Here's the drawing with two shaded views (mm, measured from the low corner). I have some questions. Coordinates: 2 decimals unless noted, no trailing zeros. Write each loop counter-clockwise with the first axis right and the second up, starting at its lowest first coordinate (ties: lowest second). Pieces come first, ordered by that corner, then holes. Notation, with made-up numbers: (7.25, -27.75) - (52.25, -27.75) arc R10 ccw to (52.25, -9.75) - close; hole circle Ø10 at (19, 87.25). An arc over 180 degrees is marked (long way). Answer in a Markdown table with one row per item. Add a question column.
Item 1: Imagine slicing it at A-A (x = 12.5). Please give me the cut outline in (y, z).
Item 2: If I drill on probe 1 along X at (y, z) = (1.5, 10); probe 2 along X at (y, z) = (4, 12.5); probe 3 along X at (y, z) = (1.25, 11.75), over which ranges is the centre line in solid material (lowest first)? Write a range as from..to.
Item 3: Imagine slicing it at C-C (z = 17.5). Please give me the cut outline in (x, y).
Item 4: We'd pull the mould along Z, two halves only. Please class the marked faces 1, 2 and 3: +Z half, -Z half, draft (parallel to the pull), parting line (faces both ways), or undercut.
Item 5: Imagine slicing it at D-D (y = 6.5). Please give me the cut outline in (x, z).
Item 6: I'm going to push a flat-ended pin straight in: pin 1 (2.5 mm diameter, centred on y = 5.5, z = 9.5, fed in from -X). Where does the tip first touch, or does it pass through?
Item 7: Imagine slicing it at B-B (z = 21.75). Please give me the cut outline in (x, y), plus the area to 3 significant figures.
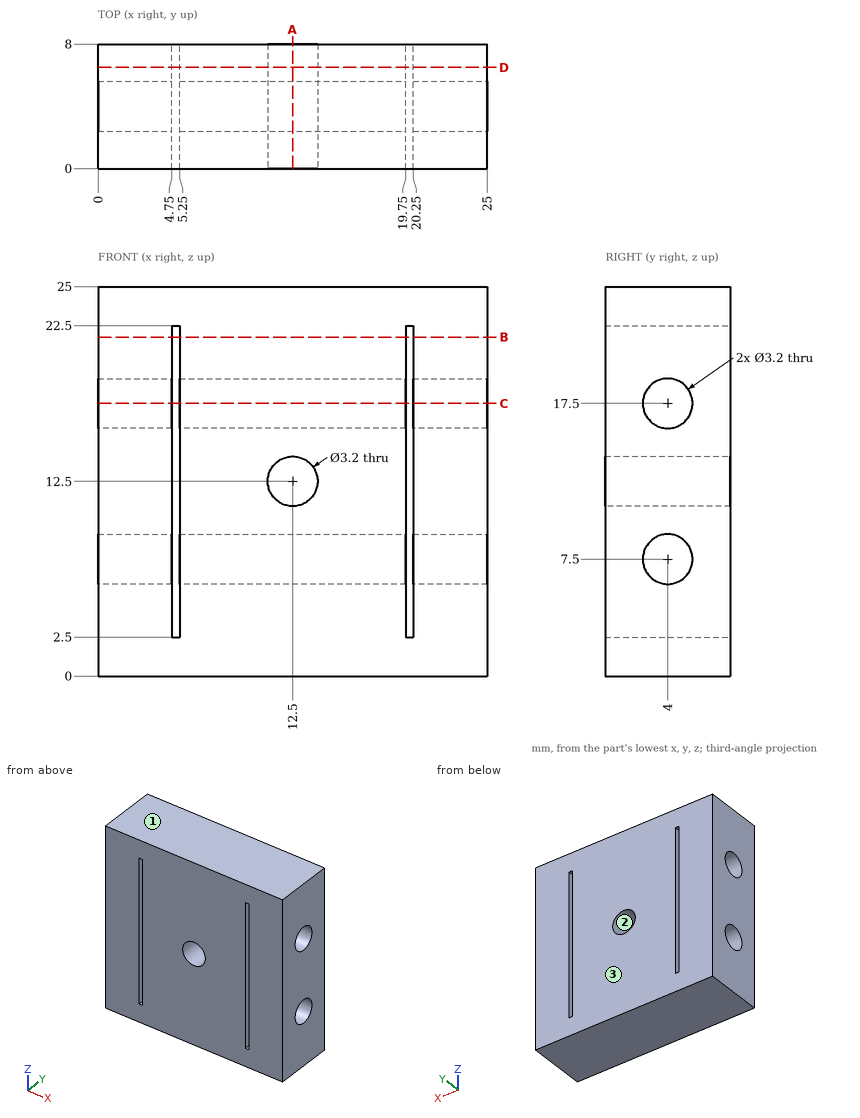
Here are the results:
| question | item | result |
|---|---|---|
| 1 | outline | (0, 0) - (8, 0) - (8, 10.9) - (0, 10.9) - close; (0, 14.1) - (8, 14.1) - (8, 25) - (0, 25) - close; hole circle Ø3.2 at (4, 7.5); hole circle Ø3.2 at (4, 17.5) |
| 2 | probe 1 | x = 0..4.75, 5.25..19.75, 20.25..25 |
| 2 | probe 2 | x = 0..4.75, 5.25..10.9, 14.1..19.75, 20.25..25 |
| 2 | probe 3 | x = 0..4.75, 5.25..11.09, 13.91..19.75, 20.25..25 |
| 3 | outline | (0, 0) - (4.75, 0) - (4.75, 2.4) - (0, 2.4) - close; (0, 5.6) - (4.75, 5.6) - (4.75, 8) - (0, 8) - close; (5.25, 0) - (19.75, 0) - (19.75, 2.4) - (5.25, 2.4) - close; (5.25, 5.6) - (19.75, 5.6) - (19.75, 8) - (5.25, 8) - close; (20.25, 0) - (25, 0) - (25, 2.4) - (20.25, 2.4) - close; (20.25, 5.6) - (25, 5.6) - (25, 8) - (20.25, 8) - close |
| 4 | face 1 | +Z half |
| 4 | face 2 | undercut |
| 4 | face 3 | draft |
| 5 | outline | (0, 0) - (25, 0) - (25, 25) - (0, 25) - close; hole (4.75, 2.5) - (5.25, 2.5) - (5.25, 22.5) - (4.75, 22.5) - close; hole circle Ø3.2 at (12.5, 12.5); hole (19.75, 2.5) - (20.25, 2.5) - (20.25, 22.5) - (19.75, 22.5) - close |
| 6 | pin 1 | stops at x = 0 |
| 7 | outline | (0, 0) - (4.75, 0) - (4.75, 8) - (0, 8) - close; (5.25, 0) - (19.75, 0) - (19.75, 8) - (5.25, 8) - close; (20.25, 0) - (25, 0) - (25, 8) - (20.25, 8) - close |
| 7 | area | 192 mm2 |
